Verification items for this drawing (mm, ordinates from the low corner). A direction names the side the tool comes from. Give positions to 0.01 mm unless a question says otherwise; leave off trailing zeros. Write each loop counter-clockwise with the first axis right and the second up, starting at its lowest first coordinate (ties: lowest second). Pieces come first, ordered by that corner, then holes. Notation, with made-up numbers: (82, -27) -> (89, -27) arc R20 cw to (89, -3) -> close; hole circle Ø9 at (12.25, 31). An arc over 180 degrees is marked (long way). Write item = value, one per line.
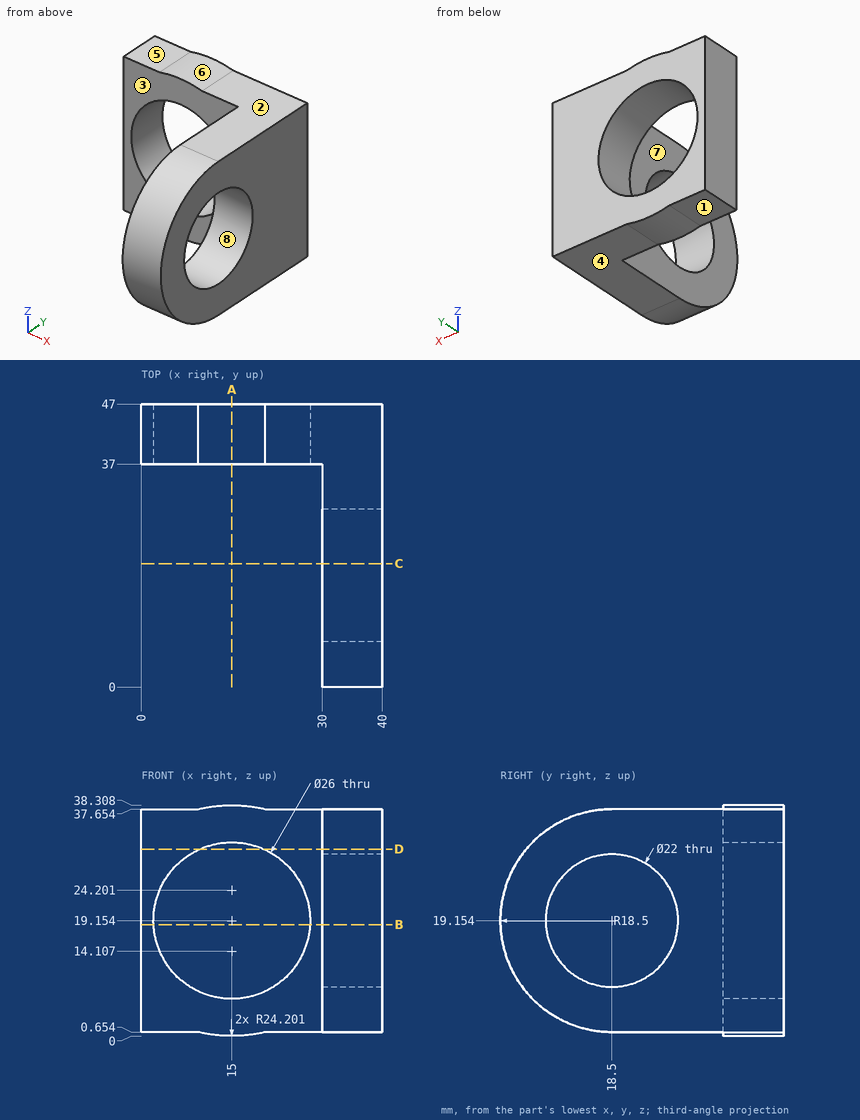
Item 1: Set-up check for the marked faces 1, 2, 3, 4 and 5: record each of +Z, -Z, +X, -X, +Y, -Y from which the full face is reachable in a straight line by a thin tool's end or side.
Response values:
face_1 = -Z, -X, +Y, -Y
face_2 = +Z, +X, +Y, -Y
face_3 = +Z, -Z, -X, -Y
face_4 = -Z, +X, +Y, -Y
face_5 = +Z, -X, +Y, -Y
Item 2: Sectioned sample at C-C on y = 20.5. Record the cut outline in (x, z), then the cut area to 3 significant figures.
Response values:
outline = (30, 0.65) -> (40, 0.65) -> (40, 8.34) -> (30, 8.34) -> close; (30, 29.97) -> (40, 29.97) -> (40, 37.65) -> (30, 37.65) -> close
area = 154 mm^2
Item 3: Mould release check, pull along Z, two halves, no side actions. Record for the marked faces 6, 7 and 8: +Z half, -Z half, draft (parallel to the pull), parting line (faces both ways), or undercut.
Response values:
face_6 = +Z half
face_7 = draft
face_8 = undercut
Item 4: Go/stop test with flat-tipped pins: P1, Ø6, axis at x = 28, y = 29.5, coming from the -Z side; P2, Ø10, axis at y = 26, z = 22, coming from the -X side; P3, Ø17.5, axis at y = 18.5, z = 19.15, coming from the +X side; P4, Ø10, axis at x = 27.5, y = 13, coming from the +Z side. Record where each tip stops, or that it passes through.
Response values:
P1 = 0.65
P2 = 30
P3 = through
P4 = 37.62
Item 5: Material ranges on line 1 (X direction, y = 12.5, z = 9.5); line 2 (X direction, y = 43.5, z = 29); line 3 (Y direction, x = 11, z = 4), recorded low to high.
Response values:
line_1 = 30 to 40
line_2 = 0 to 6.51, 23.49 to 40
line_3 = 37 to 47
Item 6: Sectioned sample at A-A on x = 15. Record the cut outline in (y, z).
Response values:
outline = (37, 0) -> (47, 0) -> (47, 6.15) -> (37, 6.15) -> close; (37, 32.15) -> (47, 32.15) -> (47, 38.31) -> (37, 38.31) -> close
Item 7: Sectioned sample at D-D on z = 31. Record the cut outline in (x, y) (1 decimal), then the cut area to 3 significant figures.
Response values:
outline = (0, 37) -> (9.6, 37) -> (9.6, 47) -> (0, 47) -> close; (20.4, 37) -> (30, 37) -> (30, 4.3) -> (40, 4.3) -> (40, 47) -> (20.4, 47) -> close
area = 620 mm^2
Item 8: Sectioned sample at B-B on z = 18.5. Record the cut outline in (x, y), then the cut area to 3 significant figures.
Response values:
outline = (0, 37) -> (2.02, 37) -> (2.02, 47) -> (0, 47) -> close; (27.98, 37) -> (30, 37) -> (30, 29.48) -> (40, 29.48) -> (40, 47) -> (27.98, 47) -> close; (30, 0.01) -> (40, 0.01) -> (40, 7.52) -> (30, 7.52) -> close
area = 291 mm^2
